from build123d import *

# Parameters (mm, degrees)
SKETCH1_W           = 50.8
SKETCH1_H           = 25.4
SKETCH1_W_2         = 44.45
SKETCH1_H_2         = 19.05
BOSS_EXTRUDE1_DEPTH = 584.2
SKETCH2_R           = 1.5875
CUT_EXTRUDE1_DEPTH  = 587.825553828
SKETCH3_R           = 3.175
CUT_EXTRUDE2_DEPTH  = 587.825553828


with BuildPart() as part:
    # Sketch1 → Boss-Extrude1 (new body)
    with BuildSketch(Plane(origin=(0, 0, 0), x_dir=(1, 0, 0), z_dir=(0, 1, 0))):
        with Locations((22.225, 9.525)):
            Rectangle(SKETCH1_W, SKETCH1_H)
        with Locations((22.225, 9.525)):
            Rectangle(SKETCH1_W_2, SKETCH1_H_2, mode=Mode.SUBTRACT)
    extrude(amount=BOSS_EXTRUDE1_DEPTH)

    # Sketch2 → Cut-Extrude1 (cut, through all)
    with BuildSketch(Plane(origin=(47.625, 0, 0), x_dir=(0, 0, -1), z_dir=(1, 0, 0))):
        with Locations((9.525, 95.25)):
            Circle(SKETCH2_R)
        with Locations((9.525, 488.95)):
            Circle(SKETCH2_R)
    extrude(amount=-CUT_EXTRUDE1_DEPTH, mode=Mode.SUBTRACT)

    # Sketch3 → Cut-Extrude2 (cut, through all)
    with BuildSketch(Plane.ZY.offset(3.175)):
        with Locations((-9.525, 25.4)):
            Circle(SKETCH3_R)
        with Locations((-9.525, 558.8)):
            Circle(SKETCH3_R)
    extrude(amount=-CUT_EXTRUDE2_DEPTH, mode=Mode.SUBTRACT)


solid = part.part
Work out the finished part from the listing and answer in its coordinate system (mm). A direction names the side the tool comes from. Give positions to 0.01 mm unless a question says otherwise; leave off trailing zeros. Loops run counter-clockwise (first coordinate to the right, second up) from the corner with the lowest first, then second, coordinate; pieces in that order, holes last. Notation, with made-up numbers: (28.25, 75) -> (78.25, 75) arc R13 ccw to (78.25, 79) -> close; hole circle Ø11 at (57.25, 71.5). An arc over 180 degrees is marked (long way). Use a Markdown table: item, result. Add a question column.
1) The part is cut by section A-A, the plane x = 5. Determine the outline of the cut face in (y, z) (3 decimals), plus the area to 3 significant figures.
2) Consider line 1 along Z through (x, y) = (42, 100) (3 decimals); line 2 along X through (y, z) = (213, -3) (3 decimals); line 3 along Z through (x, y) = (45, 558) (3 decimals). Determine where each line is inside the solid, lowest interval first.
3) The part is cut by section B-B, the plane y = 327. Determine the outline of the cut face in (x, z) (3 decimals), plus the area to 3 significant figures.
4) Which of the six approach directions +Z, -Z, +X, -X, +Y, -Y give full straight-line access (tool end or side, diameter ignored) to faces 5 (the flat face through (22, 288, 0)), 6 (the flat face through (-3.175, 288, -9))?
5) For a pull along Z with two mould halves and no side action, classify faces 1 (the flat face through (22, 288, -22.225)), 2 (the flat face through (47.625, 288, -9)), 3 (the flat face through (22, 288, 3.175)), 4 (the flat face through (0, 288, -9)) as +Z half, -Z half, draft (parallel to the pull), parting line (faces both ways), or undercut.
Reported:
| question | item | result |
|---|---|---|
| 1 | outline | (0, -22.225) -> (584.2, -22.225) -> (584.2, -19.05) -> (0, -19.05) -> close; (0, 0) -> (584.2, 0) -> (584.2, 3.175) -> (0, 3.175) -> close |
| 1 | area | 3,710 mm^2 |
| 2 | line 1 | z = -22.225 to -19.05, 0 to 3.175 |
| 2 | line 2 | x = -3.175 to 0, 44.45 to 47.625 |
| 2 | line 3 | z = -22.225 to -12.598, -6.452 to 3.175 |
| 3 | outline | (-3.175, -22.225) -> (47.625, -22.225) -> (47.625, 3.175) -> (-3.175, 3.175) -> close; hole (0, -19.05) -> (44.45, -19.05) -> (44.45, 0) -> (0, 0) -> close |
| 3 | area | 444 mm^2 |
| 4 | face 5 | +Y, -Y |
| 4 | face 6 | +Z, -Z, -X, +Y, -Y |
| 5 | face 1 | -Z half |
| 5 | face 2 | draft |
| 5 | face 3 | +Z half |
| 5 | face 4 | undercut |
